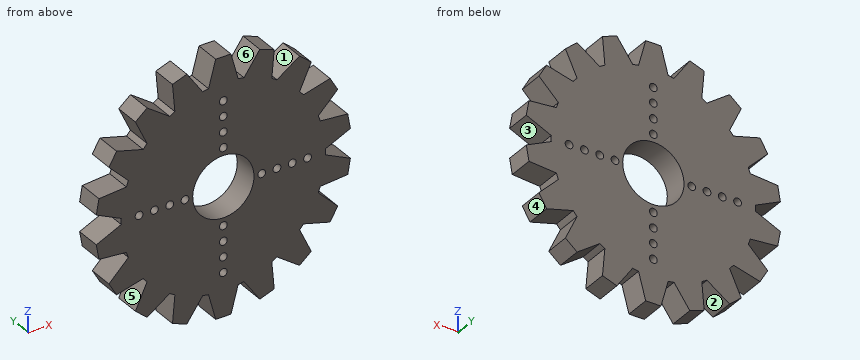
from build123d import *

# Parameters (mm, degrees)
SKETCH2_R           = 20
BOSS_EXTRUDE1_DEPTH = 5
BOSS_EXTRUDE2_DEPTH = 5
CIRPATTERN1_COUNT   = 18
SKETCH3_R           = 6
SKETCH3_R_2         = 0.762
CUT_EXTRUDE1_DEPTH  = 36.623693592
CIRPATTERN2_COUNT   = 4


with BuildPart() as part:
    # Sketch2 → Boss-Extrude1 (new body)
    with BuildSketch(Plane(origin=(0, 0, 0), x_dir=(1, 0, 0), z_dir=(0, 1, 0))):
        with Locations(Location((0, 0, 0), (0, 0, 270))):
            Circle(SKETCH2_R)
    extrude(amount=BOSS_EXTRUDE1_DEPTH)

    # Sketch2_3 → Boss-Extrude2 (add)
    with BuildSketch(Plane(origin=(0, 0, 0), x_dir=(1, 0, 0), z_dir=(0, 1, 0))):
        with BuildLine():
            ThreePointArc((-2.896233759, 19.789184673), (0, 20), (2.896233759, 19.789184673))
            Line((2.896233759, 19.789184673), (1.5, 25))
            Line((1.5, 25), (-1.5, 25))
            Line((-1.5, 25), (-2.896233759, 19.789184673))
        make_face()
    boss_extrude2 = extrude(amount=BOSS_EXTRUDE2_DEPTH)

    # CirPattern1: Boss-Extrude2 ×18 about axis
    cirpattern1_axis = Axis((0, 0, 0), (0, 1, 0))
    for i in range(1, CIRPATTERN1_COUNT):
        add(boss_extrude2.rotate(cirpattern1_axis, i * 360 / CIRPATTERN1_COUNT))

    # Sketch3 → Cut-Extrude1 (cut, through all)
    with BuildSketch(Plane(origin=(0, 0, 0), x_dir=(1, 0, 0), z_dir=(0, 1, 0))):
        with Locations(Location((0, 0, 0), (0, 0, 270))):
            Circle(SKETCH3_R)
        with Locations(Location((7.5, 0, 0), (0, 0, 270))):
            Circle(SKETCH3_R_2)
        with Locations(Location((10.5, 0, 0), (0, 0, 270))):
            Circle(SKETCH3_R_2)
        with Locations(Location((13.5, 0, 0), (0, 0, 270))):
            Circle(SKETCH3_R_2)
        with Locations(Location((16.5, 0, 0), (0, 0, 270))):
            Circle(SKETCH3_R_2)
    cut_extrude1 = extrude(amount=CUT_EXTRUDE1_DEPTH, mode=Mode.SUBTRACT)

    # CirPattern2: Cut-Extrude1 ×4 about axis
    cirpattern2_axis = Axis((0, 0, 0), (0, 1, 0))
    for i in range(1, CIRPATTERN2_COUNT):
        add(cut_extrude1.rotate(cirpattern2_axis, i * 360 / CIRPATTERN2_COUNT), mode=Mode.SUBTRACT)


solid = part.part
Geometry check sheet. Reference: the model listing, model coordinates, mm. Face numbers are marked on the shaded views. A direction names the side the tool comes from. Coordinates: 2 decimals unless noted, no trailing zeros. Order: outer loops, then holes, each group sorted by start corner. A loop starts at its lowest first (then second) coordinate and runs counter-clockwise, first axis right, second up. Notation, with made-up numbers: M 42,85 L 100,85 A25 ccw 100,101 Z; hole C -23,40 d4. An arc over 180 degrees is marked long. Use CSV: the item, a comma, the result in double quotes.
Item 1: Cross-section at B-B on z = 1.5. Record the cut outline in (x, y).
Returned:
outline,"M -21.96,0 L -5.81,0 L -5.81,5 L -21.96,5 Z; M 5.81,0 L 21.96,0 L 21.96,5 L 5.81,5 Z"
Item 2: Gauge pin test, flat end, axial feed: pin 1 Ø1 at (x, y) = (3.5, 3.5) entering from -Z. Record the tip position at first contact, or that the pin passes through.
Returned:
pin 1,"stops at z = -19.77"
Item 3: Thickness scan on line 1 along X through (y, z) = (0.5, -20); line 2 along X through (y, z) = (2.25, -19); line 3 along Z through (x, y) = (-21, 2.2). Record the ranges inside material, lowest first.
Returned:
line 1,"x = -15.06 to -14.76, -9.7 to -4.34, -2.84 to 2.84, 4.34 to 9.7, 14.76 to 15.06"
line 2,"x = -16.25 to -13.33, -9.61 to 9.61, 13.33 to 16.25"
line 3,"z = -13.63 to -9.8, -6.11 to -1.05, 1.05 to 6.11, 9.8 to 13.63"
Item 4: Tool access check on the marked faces 1, 2 and 3. Record the directions out of +Z, -Z, +X, -X, +Y, -Y that give a thin tool (end or side, any length) a straight path to the whole face; none if there is none.
Returned:
face 1,"+Z, +Y, -Y"
face 2,"-Z, +Y, -Y"
face 3,"+X, +Y, -Y"
Item 5: Cross-section at C-C on y = 3.65. Give the number of separate pieces and of enclosed holes in the cut face, then the cut area to 3 significant figures.
Returned:
separate pieces,"1"
enclosed holes,"17"
area,"1,510 mm2"
Item 6: Mould release check, pull along Z, two halves, no side actions. Record for the marked faces 4, 5 and 6: pulls with the +Z half, pulls with the -Z half, needs draft (parallel to the pull), parting line crosses it, or undercut.
Returned:
face 4,"pulls with the -Z half"
face 5,"undercut"
face 6,"pulls with the +Z half"
Item 7: Cross-section at D-D on x = 5. Record the cut outline in (y, z), then the cut area to 3 significant figures.
Returned:
outline,"M 0,-20.95 L 5,-20.95 L 5,-3.32 L 0,-3.32 Z; M 0,3.32 L 5,3.32 L 5,20.95 L 0,20.95 Z"
area,"176 mm2"
Item 8: Cross-section at A-A on x = -16.5. Record the cut outline in (y, z).
Returned:
outline,"M 0,-18.79 L 5,-18.79 L 5,-16.65 L 0,-16.65 Z; M 0,-12.62 L 5,-12.62 L 5,-0.76 L 0,-0.76 Z; M 0,0.76 L 5,0.76 L 5,12.62 L 0,12.62 Z; M 0,16.65 L 5,16.65 L 5,18.79 L 0,18.79 Z"
